Autodesk Fusion 360 part; units mm, degrees
sketch "Sketch1" plane through (0, 0, 0) normal (0, 0, 1) x (1, 0, 0)
  line L0 (0, 0) -> (122.7, 0)
  line L1 (122.7, 0) -> (122.7, 166.5)
  line L2 (122.7, 166.5) -> (0, 166.5)
  line L3 (0, 166.5) -> (0, 0)
  dimension "d1" = 166.5
  dimension "d2" = 122.7
extrude "Extrude1" add sketch "Sketch1" along normal blind 5
sketch "Sketch2" plane through (0, 0, 5) normal (0, 0, 1) x (-1, 0, 0)
  line L0 (0, -166.5) -> (0, 0)
  line L1 (0, 0) -> (-122.7, 0)
  line L2 (-122.7, 0) -> (-122.7, -166.5)
  line L3 (-122.7, -166.5) -> (0, -166.5)
  line L4 (0, -166.5) -> (-8, -166.5)
  line L5 (-8, -166.5) -> (-8, -158.5)
  line L6 (-8, -158.5) -> (0, -158.5)
  line L7 (0, -158.5) -> (0, -166.5)
  line L8 (0, 0) -> (-8, 0)
  line L9 (-8, 0) -> (-8, -8)
  line L10 (-8, -8) -> (0, -8)
  line L11 (0, -8) -> (0, 0)
  dimension "d5" = 8
  dimension "d6" = 8
  dimension "d7" = 8
  dimension "d8" = 8
extrude "Extrude2" add sketch "Sketch2" along normal blind 7 contours L0 L3 L4 L5 L6 L7 | L0 L1 L8 L9 L10 L11
ref_plane "WorkPlane1" through (61.35, 83.25, 6) normal (-1, 0, 0) x (0, -1, 0)
mirror "Mirror1" about plane through (61.35, 83.25, 6) normal (-1, 0, 0) of "Extrude2"
sketch "Sketch3" plane through (0, 0, 12) normal (0, 0, 1) x (-1, 0, 0)
  line L0 (0, -158.5) -> (-8, -158.5)
  line L1 (-8, -158.5) -> (-8, -166.5)
  line L2 (-8, -166.5) -> (0, -166.5)
  line L3 (0, -166.5) -> (0, -158.5)
  circle A0 centre (-4, -162.5) radius 1.6
  circle A1 centre (-4, -4) radius 1.6
  line L4 (-8, -8) -> (0, -8)
  line L5 (0, -8) -> (0, 0)
  dimension "d13" = 3.2
  dimension "d14" = 4
  dimension "d15" = 4
  dimension "d16" = 3.2
  dimension "d17" = 4
  dimension "d18" = 4
extrude "Extrude3" cut sketch "Sketch3" against normal blind 13 contours A0 | A1
mirror "Mirror2" about plane through (61.35, 83.25, 6) normal (-1, 0, 0) of "Extrude3"
sketch "Sketch4" plane through (0, 0, 0) normal (0, 0, -1) x (1, 0, 0)
  circle A0 centre (118.7, -4) radius 1.6
  circle A1 centre (118.7, -162.5) radius 1.6
  circle A2 centre (4, -4) radius 1.6
  circle A3 centre (4, -162.5) radius 1.6
  line L0 (0, 0) -> (0, -166.5)
  line L1 (0, -166.5) -> (122.7, -166.5)
  line L2 (122.7, -166.5) -> (122.7, 0)
  line L3 (122.7, 0) -> (0, 0)
  circle A4 centre (63.7, -28.5) radius 2.15
  circle A5 centre (112.7, -28.5) radius 2.15
  circle A6 centre (63.7, -86.5) radius 2.15
  circle A7 centre (112.7, -86.5) radius 2.15
  line L4 (60.7, -31.5) -> (66.7, -31.5)
  line L5 (66.7, -31.5) -> (66.7, -25.5)
  line L6 (66.7, -25.5) -> (60.7, -25.5)
  line L7 (60.7, -25.5) -> (60.7, -31.5)
  line L8 (109.7, -25.5) -> (115.7, -25.5)
  line L9 (115.7, -25.5) -> (115.7, -31.5)
  line L10 (115.7, -31.5) -> (109.7, -31.5)
  line L11 (109.7, -31.5) -> (109.7, -25.5)
  line L12 (60.7, -83.5) -> (66.7, -83.5)
  line L13 (66.7, -83.5) -> (66.7, -89.5)
  line L14 (66.7, -89.5) -> (60.7, -89.5)
  line L15 (60.7, -89.5) -> (60.7, -83.5)
  line L16 (109.7, -83.5) -> (115.7, -83.5)
  line L17 (115.7, -83.5) -> (115.7, -89.5)
  line L18 (115.7, -89.5) -> (109.7, -89.5)
  line L19 (109.7, -89.5) -> (109.7, -83.5)
  dimension "d23" = 4.3
  dimension "d24" = 4.3
  dimension "d25" = 4.3
  dimension "d26" = 4.3
  dimension "d27" = 49
  dimension "d28" = 58
  dimension "d29" = 10
  dimension "d30" = 80
  dimension "d39" = 6
  dimension "d40" = 6
  dimension "d41" = 3
  dimension "d42" = 3
  dimension "d43" = 3
  dimension "d44" = 3
  dimension "d45" = 6
  dimension "d46" = 6
  dimension "d47" = 6
  dimension "d48" = 6
  dimension "d49" = 3
  dimension "d51" = 6
  dimension "d52" = 6
  dimension "d53" = 3
extrude "Extrude4" cut sketch "Sketch4" against normal blind 3.3 contours A4 | A5 | A6 | A7
sketch "Sketch5" plane through (0, 0, 0) normal (0, 0, -1) x (1, 0, 0)
  circle A0 centre (118.7, -4) radius 1.6
  circle A1 centre (118.7, -162.5) radius 1.6
  circle A2 centre (4, -4) radius 1.6
  circle A3 centre (4, -162.5) radius 1.6
  line L0 (0, 0) -> (0, -166.5)
  line L1 (0, -166.5) -> (122.7, -166.5)
  line L2 (122.7, -166.5) -> (122.7, 0)
  line L3 (122.7, 0) -> (0, 0)
  circle A4 centre (4, -4) radius 2.5
  circle A5 centre (118.7, -4) radius 2.5
  circle A6 centre (118.7, -162.5) radius 2.5
  circle A7 centre (4, -162.5) radius 2.5
  circle A8 centre (63.7, -86.5) radius 2.15
  circle A9 centre (112.7, -28.5) radius 2.15
  circle A10 centre (112.7, -86.5) radius 2.15
  circle A11 centre (63.7, -28.5) radius 2.15
  dimension "d33" = 5
  dimension "d34" = 5
  dimension "d35" = 5
  dimension "d36" = 5
extrude "Extrude5" cut sketch "Sketch5" against normal blind 10 contours A4 | A5 | A6 | A7
equation "d1 = 168.3 mm - 1.8 mm"
equation "d2 = 124 mm - 1.3 mm"
Check sheet for the modelled part. Datum: model origin and axes. Units: mm. A direction names the side the tool comes from. Round coordinates to 2 decimals unless told otherwise and drop trailing zeros. Order: outer loops, then holes, each group sorted by start corner. A loop starts at its lowest first (then second) coordinate and runs counter-clockwise, first axis right, second up. Notation, with made-up numbers: (42, 28.25) -> (66, 28.25) arc R25 ccw to (66, 65.25) -> close; hole circle Ø9 at (23, 55). An arc over 180 degrees is marked (long way). Use CSV: the item, a comma, the result in double quotes.
(1) Cross-section at C-C (y = 28.5). Record the boundary of the cut face in (x, z).
Worked out:
outline,"(0, 0) -> (61.55, 0) -> (61.55, 3.3) -> (65.85, 3.3) -> (65.85, 0) -> (110.55, 0) -> (110.55, 3.3) -> (114.85, 3.3) -> (114.85, 0) -> (122.7, 0) -> (122.7, 5) -> (0, 5) -> close"
(2) Material ranges on line 1 along Y through (x, z) = (4, 11.65); line 2 along X through (y, z) = (28.5, 2.05); line 3 along Y through (x, z) = (118.5, 4.25), recorded low to high. Write a range as from..to.
Worked out:
line 1,"0..2.4, 5.6..8, 158.5..160.9, 164.1..166.5"
line 2,"0..61.55, 65.85..110.55, 114.85..122.7"
line 3,"0..1.51, 6.49..160.01, 164.99..166.5"
(3) Cross-section at D-D (y = 112). Record the boundary of the cut face in (x, z), and give its area (4 significant figures).
Worked out:
outline,"(0, 0) -> (122.7, 0) -> (122.7, 5) -> (0, 5) -> close"
area,"613.5 mm²"
(4) Cross-section at B-B (x = 112.7). Record the boundary of the cut face in (y, z), and give its area (3 significant figures).
Worked out:
outline,"(0, 0) -> (26.35, 0) -> (26.35, 3.3) -> (30.65, 3.3) -> (30.65, 0) -> (84.35, 0) -> (84.35, 3.3) -> (88.65, 3.3) -> (88.65, 0) -> (166.5, 0) -> (166.5, 5) -> (0, 5) -> close"
area,"804 mm²"
(5) Depth check by flat-ended pin: pin 1 (2 mm diameter, centred on x = 64.5, y = 87, fed in from -Z); pin 2 (4 mm diameter, centred on x = 34.5, y = 61, fed in from +Z). Enter the tip coordinate at first touch or a pass-through.
Worked out:
pin 1,"z = 3.3"
pin 2,"z = 5"
(6) Tool access check on faces 4 (the face through (110.994, 87.808, 1.627)), 5 (the face through (114.7, 4, 8)), 6 (the face through (4, 158.5, 8)), 7 (the face through (4.1, 160.7, 12)). Record the directions out of +Z, -Z, +X, -X, +Y, -Y that give a thin tool (end or side, any length) a straight path to the whole face; none if there is none.
Worked out:
face 4,"-Z"
face 5,"+Z, +Y, -Y"
face 6,"+Z, +X, -X"
face 7,"+Z, +X, -X, +Y, -Y"
(7) Cross-section at A-A (z = 7). Record the boundary of the cut face in (x, y), and give its area (3 significant figures).
Worked out:
outline,"(0, 0) -> (8, 0) -> (8, 8) -> (0, 8) -> close; (0, 158.5) -> (8, 158.5) -> (8, 166.5) -> (0, 166.5) -> close; (114.7, 0) -> (122.7, 0) -> (122.7, 8) -> (114.7, 8) -> close; (114.7, 158.5) -> (122.7, 158.5) -> (122.7, 166.5) -> (114.7, 166.5) -> close; hole circle Ø5 at (4, 4); hole circle Ø5 at (4, 162.5); hole circle Ø5 at (118.7, 4); hole circle Ø5 at (118.7, 162.5)"
area,"177 mm²"
(8) Draft check along Y on faces 1 (the face through (62, 166.5, 3)), 2 (the face through (113, 86, 3.3)), 3 (the face through (122.7, 82, 3)). Enter one of: pulls with the +Y half, pulls with the -Y half, needs draft (parallel to the pull), parting line crosses it, or undercut.
Worked out:
face 1,"pulls with the +Y half"
face 2,"undercut"
face 3,"needs draft"
